Read the model definition and answer for the solid it produces. Units are mm, in the model's axes. Give positions to 0.01 mm unless a question says otherwise; leave off trailing zeros. Order: outer loops, then holes, each group sorted by start corner. A loop starts at its lowest first (then second) coordinate and runs counter-clockwise, first axis right, second up. Notation, with made-up numbers: (37.5, -13.75) -> (65.5, -13.75) arc R27 cw to (65.5, 4.25) -> close; hole circle Ø1 at (-7, 28). An arc over 180 degrees is marked (long way). Answer as CSV lines item,"result". Start each with the question number.
1) A flat-ended cylindrical pin translates along its axis: pin 1 Ø5.5 at (x, z) = (24.75, 24.75) entering from -Y. Find the tip coordinate at first contact, or state that the pin passes through.
2) Find section C-C (y = -0.2). State how many separate pieces and enclosed holes the cut face has, and give its area (3 significant figures).
3) Straight lines are drawn through the part: L1, parallel to Z at x = 0, y = -0.4; L2, parallel to Z at x = -24.5, y = -0.15; L3, parallel to X at y = -0.55, z = -25.5. For each, find the intervals that lie inside material, in ascending order. Write a range as from..to.
4) The mould has two halves that part along Z. Classify faces 1 (the face through (22.97, -0.51, -27.53)), 2 (the face through (18, 0, -18)), 3 (the face through (40.06, -0.49, 12.62)), 4 (the face through (-21.452, -0.507, 24.604)): +Z half, -Z half, draft (parallel to the pull), parting line (faces both ways), or undercut.
5) Find section B-B (z = 6.5). Determine the outline of the cut face in (x, y), and give its area (3 significant figures).
6) Find section D-D (z = 26.5). Determine the outline of the cut face in (x, y), and give its area (3 significant figures).
7) Find section A-A (x = -26). Determine the outline of the cut face in (y, z), and give its area (3 significant figures).
```python
from build123d import *

# Parameters (mm, degrees)
F0_R     = 42
F0_R_2   = 3.3
F0_R_3   = 24
F1_DEPTH = 1
F2_D     = 6.6


with BuildPart() as f1:
    # F0 (on Front) → F1 (new body)
    with BuildSketch(Plane.XZ):
        Circle(F0_R)
        with Locations((-24.7487373415, -24.7487373415)):
            Circle(F0_R_2, mode=Mode.SUBTRACT)
        with Locations((0, -34.2780984938)):
            Circle(F0_R_2, mode=Mode.SUBTRACT)
        with Locations((24.7487373415, -24.7487373415)):
            Circle(F0_R_2, mode=Mode.SUBTRACT)
        with Locations((-35, 0)):
            Circle(F0_R_2, mode=Mode.SUBTRACT)
        with Locations((-24.7487373415, 24.7487373415)):
            Circle(F0_R_2, mode=Mode.SUBTRACT)
        Circle(F0_R_3, mode=Mode.SUBTRACT)
        with Locations((35, 0)):
            Circle(F0_R_2, mode=Mode.SUBTRACT)
        with Locations((0, 35)):
            Circle(F0_R_2, mode=Mode.SUBTRACT)
        with Locations((24.7487373415, 24.7487373415)):
            Circle(F0_R_2, mode=Mode.SUBTRACT)
        with Locations((0, 35)):
            Circle(F0_R_2)
        with Locations((-24.7487373415, 24.7487373415)):
            Circle(F0_R_2)
        with Locations((-24.7487373415, -24.7487373415)):
            Circle(F0_R_2)
        with Locations((-35, 0)):
            Circle(F0_R_2)
        with Locations((0, -34.2780984938)):
            Circle(F0_R_2)
        with Locations((24.7487373415, -24.7487373415)):
            Circle(F0_R_2)
        with Locations((35, 0)):
            Circle(F0_R_2)
        with Locations((24.7487373415, 24.7487373415)):
            Circle(F0_R_2)
    extrude(amount=F1_DEPTH)

    # F2 (through all)
    with Locations(Plane(origin=(0, 0, 0), x_dir=(1, 0, 0), z_dir=(0, 1, 0))):
        with Locations((24.7487373415, -24.7487373415), (35, 0), (24.7487373415, 24.7487373415), (0, 34.2780984938), (-24.7487373415, 24.7487373415), (-35, 0), (-24.7487373415, -24.7487373415), (0, -35)):
            Hole(F2_D / 2)


solid = f1.part
```
Findings below:
1,pin 1,"through"
2,separate pieces,"1"
2,enclosed holes,"9"
2,area,"3,460 mm²"
3,L1,"-42..-37.58, -30.98..-24, 24..31.7, 38.3..42"
3,L2,"-34.11..-28.04, -21.46..21.46, 28.04..34.11"
3,L3,"-33.37..-27.96, -21.54..21.54, 27.96..33.37"
4,face 1,"undercut"
4,face 2,"draft"
4,face 3,"parting line"
4,face 4,"undercut"
5,outline,"(-41.49, -1) -> (-23.1, -1) -> (-23.1, 0) -> (-41.49, 0) -> close; (23.1, -1) -> (41.49, -1) -> (41.49, 0) -> (23.1, 0) -> close"
5,area,"36.8 mm²"
6,outline,"(-32.58, -1) -> (-27.55, -1) -> (-27.55, 0) -> (-32.58, 0) -> close; (-21.95, -1) -> (21.95, -1) -> (21.95, 0) -> (-21.95, 0) -> close; (27.55, -1) -> (32.58, -1) -> (32.58, 0) -> (27.55, 0) -> close"
6,area,"54.0 mm²"
7,outline,"(-1, -32.98) -> (0, -32.98) -> (0, -27.8) -> (-1, -27.8) -> close; (-1, -21.7) -> (0, -21.7) -> (0, 21.7) -> (-1, 21.7) -> close; (-1, 27.8) -> (0, 27.8) -> (0, 32.98) -> (-1, 32.98) -> close"
7,area,"53.8 mm²"
